Verification items for the finished model (mm, model axes). Face numbers are marked on the shaded views. Coordinates: 2 decimals unless noted, no trailing zeros. Write each loop counter-clockwise with the first axis right and the second up, starting at its lowest first coordinate (ties: lowest second). Pieces come first, ordered by that corner, then holes. Notation, with made-up numbers: M 45,56 L 60,56 A8 cw 60,65 Z; hole C -6,73 d3. An arc over 180 degrees is marked long. One line per item, written item: value.
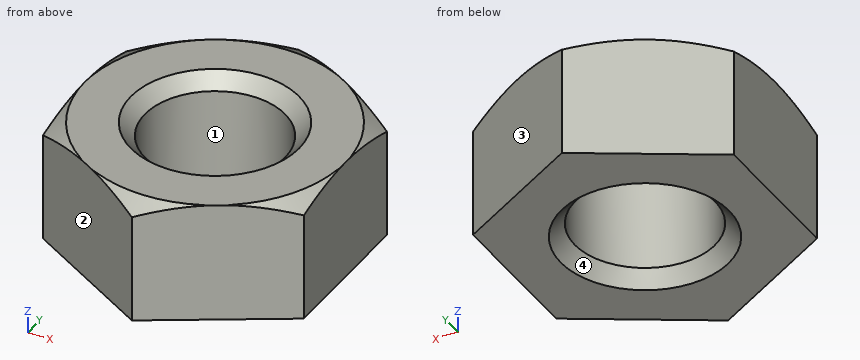
```python
from build123d import *

# Parameters (mm, degrees)
F1_DEPTH = 6
F2_R     = 3.5
F3_DEPTH = 6.001
F6_SIZE  = 0.7


with BuildPart() as f1:
    # F0 (on Top) → F1 (new body)
    with BuildSketch(Plane.XY):
        Polygon((6.5, -3.752777), (6.5, 3.752777), (0, 7.505553), (-6.5, 3.752777), (-6.5, -3.752777), (0, -7.505553), align=None)
    extrude(amount=F1_DEPTH)

    # F2 (on face) → F3 (cut, through all)
    with BuildSketch(Plane.XY.offset(6)):
        Circle(F2_R)
    extrude(amount=-F3_DEPTH, mode=Mode.SUBTRACT)

    # F4 (on Front) → F5 (revolve, cut)
    with BuildSketch(Plane.XZ):
        Polygon((10.708706, 6), (6.5, 6), (10.708706, 3.570103), align=None)
    revolve(axis=Axis((0, 0, 2.326309), (0, 0, 1)), mode=Mode.SUBTRACT)

    # F6
    f6_edges = [f1.edges().sort_by_distance(p)[0] for p in [
        (-3.5, 0, 6),
        (-3.5, 0, 0),
    ]]
    chamfer(f6_edges, length=F6_SIZE)


solid = f1.part
```
Item 1: Draft check along Y on the marked faces 1, 2, 3 and 4. Enter one of: released by +Y, released by -Y, zero draft, split by the parting line, or undercut.
The answers:
face 1: undercut
face 2: released by -Y
face 3: released by +Y
face 4: undercut
Item 2: Cross-section at A-A, the plane z = 2.8. Enter the section's corners in (x, y), and give its area (3 significant figures).
The answers:
outline: M -6.5,-3.75 L 0,-7.51 L 6.5,-3.75 L 6.5,3.75 L 0,7.51 L -6.5,3.75 Z; hole C 0,0 d7
area: 108 mm²
Item 3: Scan lines: line 1 (X direction, y = 2.75, z = 2.45); line 2 (Y direction, x = 2.5, z = 3.8); line 3 (X direction, y = 1.5, z = 5.4). Record each from-to range of solid material in increasing order.
The answers:
line 1: x = -6.5 to -2.17, 2.17 to 6.5
line 2: y = -6.06 to -2.45, 2.45 to 6.06
line 3: x = -6.5 to -3.27, 3.27 to 6.5
Item 4: Go/stop test with flat-tipped pins: P1, Ø3, axis at x = 3.5, z = 2, coming from the -Y side; P2, Ø2, axis at x = -2.5, z = 5, coming from the -Y side. Record where each tip stops, or that it passes through.
The answers:
P1: stops at y = -6.35
P2: stops at y = -6.64
